Autodesk Inventor part; units mm, degrees
ref_plane "YZ Plane" through (0, 0, 0) normal (1, 0, 0) x (0, 1, 0)
ref_plane "XZ Plane" through (0, 0, 0) normal (0, 1, 0) x (-1, 0, 0)
ref_plane "XY Plane" through (0, 0, 0) normal (0, 0, 1) x (1, 0, 0)
sketch "Sketch1" plane through (0, 0, 0) normal (0, 0, 1) x (1, 0, 0)
  line L0 (-20, -20) -> (20, -20)
  line L1 (20, -20) -> (20, 20)
  line L2 (20, 20) -> (-20, 20)
  line L3 (-20, 20) -> (-20, -20)
  line L4 (-20, -20) -> (20, 20) construction
  line L5 (20, -20) -> (-20, 20) construction
  point P0 (0, 0)
  dimension "d0" = 40
  dimension "d1" = 40
extrude "Extrusion1" add sketch "Sketch1" along normal blind 1.5
sketch "Sketch2" plane through (0, 0, 1.5) normal (0, 0, 1) x (1, 0, 0)
  line L0 (-28, 0) -> (28, 0)
  line L1 (-18, -6) -> (-10.5, -6)
  line L2 (-10.5, -6) -> (-10.5, 6)
  line L3 (-10.5, 6) -> (-18, 6)
  line L4 (-18, 6) -> (-18, -6)
  line L5 (-18, -6) -> (-10.5, 6) construction
  line L6 (-10.5, -6) -> (-18, 6) construction
  line L7 (-20, 20) -> (-20, -20)
  point P0 (0, 0)
  point P1 (-14.25, 0)
  dimension "d4" = 7.5
  dimension "d5" = 12
  dimension "d6" = 2
extrude "Extrusion2" add sketch "Sketch2" along normal blind 5
sketch "Sketch3" plane through (0, 0, 1.5) normal (0, 0, 1) x (1, 0, 0)
  line L0 (16, -15) -> (-4, -15)
  line L1 (-4, -15) -> (-4, 5)
  line L2 (-4, 5) -> (16, 5)
  line L3 (16, 5) -> (16, -15)
  line L4 (20, -20) -> (20, 20)
  line L5 (-20, -20) -> (20, -20)
  point P0 (0, 0)
  dimension "d9" = 4
  dimension "d10" = 5
  dimension "d11" = 20
  dimension "d12" = 20
extrude "Extrusion3" add sketch "Sketch3" along normal blind 5
sketch "Sketch4" plane through (-18, -6, 1.5) normal (-1, 0, 0) x (0, 0, 1)
  circle A0 centre (2.533, 9.2518) radius 1.0325
  circle A1 centre (2.533, 5.4062) radius 1.0614
  circle A2 centre (2.3673, 1.4611) radius 1.0614
  point P0 (-1.5, 6)
extrude "Extrusion4" add sketch "Sketch4" along normal blind 5
properties part number "oledlcd"
Can you work these out from the model? Positions are in its coordinate system, mm. A direction names the side the tool comes from. Round coordinates to 2 decimals unless told otherwise and drop trailing zeros. Loops run counter-clockwise (first coordinate to the right, second up) from the corner with the lowest first, then second, coordinate; pieces in that order, holes last. Notation, with made-up numbers: M -28,22.5 L -18,22.5 A23 cw -18,45.5 Z; hole C 23,31.25 d6. An arc over 180 degrees is marked long. Write item = value, one per line. Start each with the question number.
(1) Suppose I cut it at D-D on y = 1. Write out the boundary of the cut face in (x, z), plus the area to 4 significant figures.
(2) If we mould it in two halves opening along Y, with no side actions, what happens to faces 5 (the face through (6, -15, 4)), 6 (the face through (-20.46, 4.26, 3.81)), 7 (the face through (16, -5, 4))? For each: released by +Y, released by -Y, zero draft, split by the parting line, or undercut.
(3) I'm going to push flat-ended pins straight in: P1, Ø2.5, axis at y = -7, z = 4.5, coming from the +X side; P2, Ø2.5, axis at x = 3, z = 3.5, coming from the -Y side; P3, Ø1.5, axis at x = -14.5, z = 3, coming from the +Y side. Where does each tip first touch, or does it pass through?
(4) I need wall thicknesses on line 1 along X through (y, z) = (1.5, 4.25); line 2 along X through (y, z) = (4, 4); line 3 along Z through (x, y) = (-7, -5). Which ranges of each line are inside material? Lowest first, please.
(5) Suppose I cut it at B-B on x = -16. Write out the boundary of the cut face in (y, z).
(6) Suppose I cut it at A-A on z = 2. Write out the boundary of the cut face in (x, y), plus the area to 3 significant figures.
(7) Which directions (+Z, -Z, +X, -X, +Y, -Y) give clear straight access to the entire face, cutting with the end or side of a thin tool? Please do faces 1 (the face through (-10.5, 0, 4)), 2 (the face through (-14, -6, 4)), 3 (the face through (-14, 6, 4)), 4 (the face through (-20.465, -0.913, 5.045)).
(8) Suppose I cut it at C-C on y = -10. Write out the boundary of the cut face in (x, z), plus the area to 3 significant figures.
Answer block:
q1.outline = M -20,0 L 20,0 L 20,1.5 L 16,1.5 L 16,6.5 L -4,6.5 L -4,1.5 L -10.5,1.5 L -10.5,6.5 L -18,6.5 L -18,1.5 L -20,1.5 Z
q1.area = 197.5 mm²
q2.face_5 = released by -Y
q2.face_6 = undercut
q2.face_7 = zero draft
q3.P1 = 16
q3.P2 = -15
q3.P3 = 6
q4.line_1 = -18 to -10.5, -4 to 16
q4.line_2 = -23 to -10.5, -4 to 16
q4.line_3 = 0 to 1.5
q5.outline = M -20,0 L 20,0 L 20,1.5 L 6,1.5 L 6,6.5 L -6,6.5 L -6,1.5 L -20,1.5 Z
q6.outline = M -18,-6 L -10.5,-6 L -10.5,6 L -18,6 Z; M -4,-15 L 16,-15 L 16,5 L -4,5 Z
q6.area = 490 mm²
q7.face_1 = +Z, +Y, -Y
q7.face_2 = +Z, -X, -Y
q7.face_3 = +Z, +X, -X, +Y
q7.face_4 = -X
q8.outline = M -20,0 L 20,0 L 20,1.5 L 16,1.5 L 16,6.5 L -4,6.5 L -4,1.5 L -20,1.5 Z
q8.area = 160 mm²
